Source: three-view drawing plus pictorial views. Frame: mm from the lowest corner of the part. Coordinates: 2 decimals unless noted, no trailing zeros. Write each loop counter-clockwise with the first axis right and the second up, starting at its lowest first coordinate (ties: lowest second). Pieces come first, ordered by that corner, then holes. Notation, with made-up numbers: (-9.5, -28) -> (16.5, -28) arc R10 ccw to (16.5, -9) -> close; hole circle Ø4 at (42.5, -10). An arc over 180 degrees is marked (long way). One line per item, written item: value. Start each with the question number.
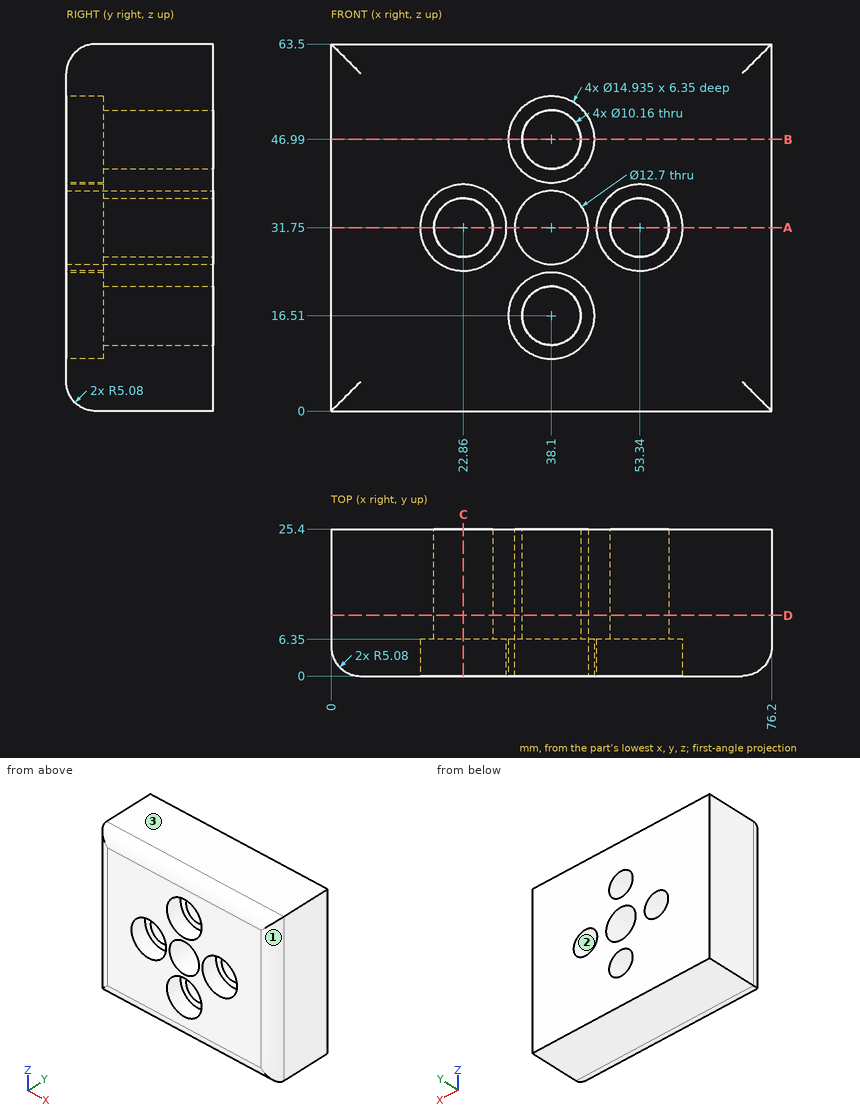
Q1. Draft query along X for the marked faces 1, 2 and 3. Return one class per face: pulls with the +X half, pulls with the -X half, needs draft (parallel to the pull), parting line crosses it, or undercut.
Q2. Cut plane B-B on z = 46.99. Output: boundary loops of the cut face in (x, y).
Q3. Cut plane D-D on y = 10.5. Output: boundary loops of the cut face in (x, z).
Q4. Line query: L1, parallel to X at y = 9.5, z = 32 (1 decimal); L2, parallel to Z at x = 53.34, y = 4.75; L3, parallel to Z at x = 38.1, y = 3.5. Output: solid intervals per line, ascending. Write a range as from..to.
Q5. Cut plane C-C on x = 22.86. Output: boundary loops of the cut face in (y, z), and give its area (3 significant figures).
Q6. Cut plane A-A on z = 31.75. Output: boundary loops of the cut face in (x, y).
Q7. First-contact query: P1, Ø10, axis at x = 39.5, z = 11, coming from the -Y side; P2, Ø7.5, axis at x = 36.5, z = 47.5, coming from the -Y side. Flat tips, straight axial feed; report the tip coordinate or a pass-through.
Solution:
1. face 1: pulls with the +X half
1. face 2: undercut
1. face 3: needs draft
2. outline: (0, 5.08) arc R5.08 ccw to (5.08, 0) -> (30.63, 0) -> (30.63, 6.35) -> (33.02, 6.35) -> (33.02, 25.4) -> (0, 25.4) -> close; (43.18, 6.35) -> (45.57, 6.35) -> (45.57, 0) -> (71.12, 0) arc R5.08 ccw to (76.2, 5.08) -> (76.2, 25.4) -> (43.18, 25.4) -> close
3. outline: (0, 0) -> (76.2, 0) -> (76.2, 63.5) -> (0, 63.5) -> close; hole circle Ø10.16 at (22.86, 31.75); hole circle Ø12.7 at (38.1, 31.75); hole circle Ø10.16 at (38.1, 16.51); hole circle Ø10.16 at (38.1, 46.99); hole circle Ø10.16 at (53.34, 31.75)
4. L1: 0..17.8, 27.9..31.8, 44.4..48.3, 58.4..76.2
4. L2: 0.01..24.28, 39.22..63.49
4. L3: 0.25..9.04, 23.98..25.4, 38.1..39.52, 54.46..63.25
5. outline: (0, 5.08) arc R5.08 ccw to (5.08, 0) -> (25.4, 0) -> (25.4, 26.67) -> (6.35, 26.67) -> (6.35, 24.28) -> (0, 24.28) -> close; (0, 39.22) -> (6.35, 39.22) -> (6.35, 36.83) -> (25.4, 36.83) -> (25.4, 63.5) -> (5.08, 63.5) arc R5.08 ccw to (0, 58.42) -> close
5. area: 1,310 mm²
6. outline: (0, 5.08) arc R5.08 ccw to (5.08, 0) -> (15.39, 0) -> (15.39, 6.35) -> (17.78, 6.35) -> (17.78, 25.4) -> (0, 25.4) -> close; (27.94, 6.35) -> (30.33, 6.35) -> (30.33, 0) -> (31.75, 0) -> (31.75, 25.4) -> (27.94, 25.4) -> close; (44.45, 0) -> (45.87, 0) -> (45.87, 6.35) -> (48.26, 6.35) -> (48.26, 25.4) -> (44.45, 25.4) -> close; (58.42, 6.35) -> (60.81, 6.35) -> (60.81, 0) -> (71.12, 0) arc R5.08 ccw to (76.2, 5.08) -> (76.2, 25.4) -> (58.42, 25.4) -> close
7. P1: y = 0
7. P2: y = 6.35
